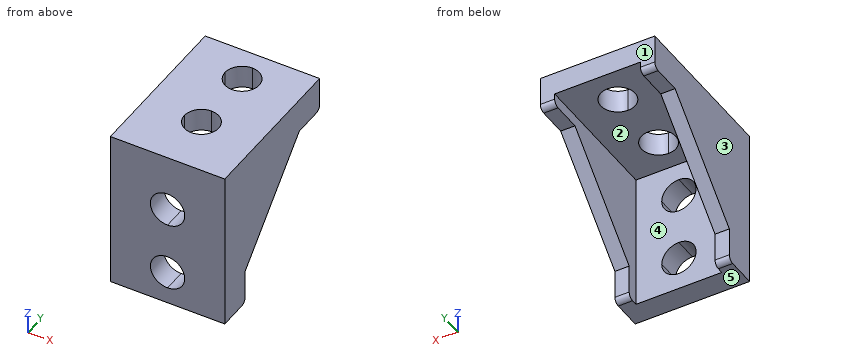
```python
from build123d import *

# Parameters (mm, degrees)
SKETCH1_W               = 17.5
SKETCH1_H               = 16
BOSS_EXTRUDE1_DEPTH     = 6
SKETCH2_W               = 2.5
SKETCH2_H               = 16
BOSS_EXTRUDE2_DEPTH     = 22
BOSS_EXTRUDE3_DEPTH     = 2.5
BOSS_EXTRUDE4_DEPTH     = 6
SKETCH5_W               = 20
SKETCH5_H               = 28
BOSS_EXTRUDE5_DEPTH     = 6
CUT_EXTRUDE1_REACH      = 40.21
SKETCH7_W               = 15
SKETCH7_H               = 22
CUT_EXTRUDE2_REACH      = 40.21
SKETCH9_W               = 15
SKETCH9_H               = 24
CUT_EXTRUDE3_DEPTH      = 45.362146026
CUT_EXTRUDE4_DEPTH      = 39.209946349
CUT_EXTRUDE5_DEPTH      = 41.841155713
BOSS_EXTRUDE6_DEPTH     = 6
BOSS_EXTRUDE7_DEPTH     = 6
BOSS_EXTRUDE8_DEPTH     = 6
BOSS_EXTRUDE9_DEPTH     = 6
FILLET1_R               = 1
SKETCH17_W              = 15
SKETCH17_H              = 24
BOSS_EXTRUDE10_DEPTH    = 4
SKETCH18_W              = 15
SKETCH18_H              = 24
BOSS_EXTRUDE11_DEPTH    = 4
CUT_EXTRUDE6_DEPTH      = 10
CUT_EXTRUDE7_DEPTH      = 10
CUT_EXTRUDE8_DEPTH      = 39.52596527
CUT_EXTRUDE8_DEPTH_BACK = 39.52596527
SKETCH21_W              = 6
SKETCH21_H              = 1.6
CUT_EXTRUDE9_DEPTH      = 39.52596527
CUT_EXTRUDE9_DEPTH_BACK = 39.52596527
SKETCH22_W              = 6
SKETCH22_H              = 1.6


with BuildPart() as part:
    # Sketch1 → Boss-Extrude1 (new body)
    with BuildSketch(Plane.XY):
        with Locations((-1.25, 14)):
            Rectangle(SKETCH1_W, SKETCH1_H)
    extrude(amount=-BOSS_EXTRUDE1_DEPTH)

    # Sketch2 → Boss-Extrude2 (add)
    with BuildSketch(Plane(origin=(0, 0, -6), x_dir=(-1, 0, 0), z_dir=(0, 0, -1))):
        with Locations((8.75, 14)):
            Rectangle(SKETCH2_W, SKETCH2_H)
    extrude(amount=BOSS_EXTRUDE2_DEPTH)

    # Sketch3 → Boss-Extrude3 (add)
    with BuildSketch(Plane(origin=(7.5, 0, 0), x_dir=(0, 0, -1), z_dir=(1, 0, 0))):
        Polygon((6, 22), (22, 6), (0, 6), (0, 22), align=None)
    extrude(amount=BOSS_EXTRUDE3_DEPTH)

    # Sketch4 → Boss-Extrude4 (add)
    with BuildSketch(Plane(origin=(0, 22, 0), x_dir=(-1, 0, 0), z_dir=(0, 1, 0))):
        Polygon((7.5, -6), (-10, -6), (-10, 0), (10, 0), (10, -28), (7.5, -28), align=None)
    extrude(amount=BOSS_EXTRUDE4_DEPTH)

    # Sketch5 → Boss-Extrude5 (add)
    with BuildSketch(Plane.XZ.offset(-6)):
        with Locations((0, -14)):
            Rectangle(SKETCH5_W, SKETCH5_H)
    extrude(amount=BOSS_EXTRUDE5_DEPTH)

    # Sketch7 → Cut-Extrude1 (cut, up to next)
    with BuildSketch(Plane.XY.offset(-4), mode=Mode.PRIVATE) as cut_extrude1_sk1:
        with Locations((0, 17)):
            Rectangle(SKETCH7_W, SKETCH7_H)
    cut_extrude1_tool1 = extrude(cut_extrude1_sk1.sketch, amount=-CUT_EXTRUDE1_REACH, mode=Mode.PRIVATE) & part.part
    add(cut_extrude1_tool1.solids().sort_by_distance((0, 17, -4))[0], mode=Mode.SUBTRACT)

    # Sketch9 → Cut-Extrude2 (cut, up to next)
    with BuildSketch(Plane.XZ.offset(-4), mode=Mode.PRIVATE) as cut_extrude2_sk1:
        with Locations((0, -16)):
            Rectangle(SKETCH9_W, SKETCH9_H)
    cut_extrude2_tool1 = extrude(cut_extrude2_sk1.sketch, amount=-CUT_EXTRUDE2_REACH, mode=Mode.PRIVATE) & part.part
    add(cut_extrude2_tool1.solids().sort_by_distance((0, 4, -16))[0], mode=Mode.SUBTRACT)

    # Sketch10 → Cut-Extrude3 (cut, through all)
    with BuildSketch(Plane.ZY.offset(10)):
        Polygon((-28, 28), (-28, 6), (-22, 6), (-6, 22), (-6, 28), align=None)
    extrude(amount=-CUT_EXTRUDE3_DEPTH, mode=Mode.SUBTRACT)

    # Sketch11 → Cut-Extrude4 (cut, through all)
    with BuildSketch(Plane(origin=(0, 0, -4), x_dir=(-1, 0, 0), z_dir=(0, 0, -1))):
        with BuildLine():
            Line((3.25, 12.5), (3.25, 18))
            ThreePointArc((3.25, 18), (0, 21.25), (-3.25, 18))
            Line((-3.25, 18), (-3.25, 12.5))
            ThreePointArc((-3.25, 12.5), (0, 9.25), (3.25, 12.5))
        make_face()
    extrude(amount=-CUT_EXTRUDE4_DEPTH, mode=Mode.SUBTRACT)

    # Sketch12 → Cut-Extrude5 (cut, through all)
    with BuildSketch(Plane.XZ):
        with BuildLine():
            Line((3.25, -18), (3.25, -12.5))
            ThreePointArc((3.25, -12.5), (0, -9.25), (-3.25, -12.5))
            Line((-3.25, -12.5), (-3.25, -18))
            ThreePointArc((-3.25, -18), (0, -21.25), (3.25, -18))
        make_face()
    extrude(amount=-CUT_EXTRUDE5_DEPTH, mode=Mode.SUBTRACT)

    # Sketch13 → Boss-Extrude6 (add)
    with BuildSketch(Plane(origin=(3, 0, 0), x_dir=(0, 0, -1), z_dir=(1, 0, 0))):
        Polygon((0, 26.5), (-1.6, 24.9), (-1.6, 23.5), (0, 23.5), align=None)
    extrude(amount=-BOSS_EXTRUDE6_DEPTH)

    # Sketch14 → Boss-Extrude7 (add)
    with BuildSketch(Plane(origin=(3, 0, 0), x_dir=(0, 0, -1), z_dir=(1, 0, 0))):
        Polygon((0, 6.5), (-1.6, 4.9), (-1.6, 3.5), (0, 3.5), align=None)
    extrude(amount=-BOSS_EXTRUDE7_DEPTH)

    # Sketch15 → Boss-Extrude8 (add)
    with BuildSketch(Plane(origin=(3, 0, 0), x_dir=(0, 0, -1), z_dir=(1, 0, 0))):
        Polygon((23.5, 0), (23.5, -1.6), (24.9, -1.6), (26.5, 0), align=None)
    extrude(amount=-BOSS_EXTRUDE8_DEPTH)

    # Sketch16 → Boss-Extrude9 (add)
    with BuildSketch(Plane(origin=(3, 0, 0), x_dir=(0, 0, -1), z_dir=(1, 0, 0))):
        Polygon((3.5, 0), (3.5, -1.6), (4.9, -1.6), (6.5, 0), align=None)
    extrude(amount=-BOSS_EXTRUDE9_DEPTH)

    # Fillet1
    fillet1_edges = [part.edges().sort_by_distance(p)[0] for p in [
        (-8.75, 6, -28),
        (8.75, 28, -6),
        (8.75, 6, -28),
        (-8.75, 28, -6),
    ]]
    fillet(fillet1_edges, radius=FILLET1_R)

    # Sketch17 → Boss-Extrude10 (add)
    with BuildSketch(Plane(origin=(0, 4, 0), x_dir=(1, 0, 0), z_dir=(0, 1, 0))):
        with Locations((0, 16)):
            Rectangle(SKETCH17_W, SKETCH17_H)
    extrude(amount=-BOSS_EXTRUDE10_DEPTH)

    # Sketch18 → Boss-Extrude11 (add)
    with BuildSketch(Plane(origin=(0, 0, -4), x_dir=(-1, 0, 0), z_dir=(0, 0, -1))):
        with Locations((0, 16)):
            Rectangle(SKETCH18_W, SKETCH18_H)
    extrude(amount=-BOSS_EXTRUDE11_DEPTH)

    # Sketch20 → Cut-Extrude6 (cut)
    with BuildSketch(Plane(origin=(0, 0, -4), x_dir=(-1, 0, 0), z_dir=(0, 0, -1))):
        with BuildLine():
            ThreePointArc((3, 22), (2.121320344, 24.121320344), (0, 25))
            Line((0, 25), (0, 22))
            Line((0, 22), (0, 19))
            ThreePointArc((0, 19), (2.121320344, 19.878679656), (3, 22))
        make_face()
        with BuildLine():
            Line((0, 22), (0, 25))
            ThreePointArc((0, 25), (-3, 22), (0, 19))
            Line((0, 19), (0, 22))
        make_face()
        with BuildLine():
            ThreePointArc((3, 10), (2.121320344, 12.121320344), (0, 13))
            Line((0, 13), (0, 10))
            Line((0, 10), (0, 7))
            ThreePointArc((0, 7), (2.121320344, 7.878679656), (3, 10))
        make_face()
        with BuildLine():
            Line((0, 10), (0, 13))
            ThreePointArc((0, 13), (-3, 10), (0, 7))
            Line((0, 7), (0, 10))
        make_face()
    extrude(amount=-CUT_EXTRUDE6_DEPTH, mode=Mode.SUBTRACT)

    # Sketch19 → Cut-Extrude7 (cut)
    with BuildSketch(Plane(origin=(0, 4, 0), x_dir=(1, 0, 0), z_dir=(0, 1, 0))):
        with BuildLine():
            Line((0, 19.123546409), (0, 22))
            Line((0, 22), (0, 22.123546409))
            Line((0, 22.123546409), (0, 25.123546409))
            ThreePointArc((0, 25.123546409), (-3, 22.123546409), (0, 19.123546409))
        make_face()
        with BuildLine():
            Line((0, 22.123546409), (0, 22))
            Line((0, 22), (0, 19.123546409))
            ThreePointArc((0, 19.123546409), (2.121320344, 20.002226065), (3, 22.123546409))
            ThreePointArc((3, 22.123546409), (2.121320344, 24.244866752), (0, 25.123546409))
            Line((0, 25.123546409), (0, 22.123546409))
        make_face()
        with BuildLine():
            ThreePointArc((3, 10), (2.121320344, 12.121320344), (0, 13))
            Line((0, 13), (0, 10))
            Line((0, 10), (0, 7))
            ThreePointArc((0, 7), (2.121320344, 7.878679656), (3, 10))
        make_face()
        with BuildLine():
            Line((0, 10), (0, 13))
            ThreePointArc((0, 13), (-3, 10), (0, 7))
            Line((0, 7), (0, 10))
        make_face()
    extrude(amount=-CUT_EXTRUDE7_DEPTH, mode=Mode.SUBTRACT)

    # Sketch21 → Cut-Extrude8 (cut, two sides: drawn at the far end of the back side and taken through both)
    with BuildSketch(Plane.XZ.offset(-3.5).offset(-CUT_EXTRUDE8_DEPTH_BACK)):
        with Locations((0, 0.8)):
            Rectangle(SKETCH21_W, SKETCH21_H)
    extrude(amount=CUT_EXTRUDE8_DEPTH + CUT_EXTRUDE8_DEPTH_BACK, mode=Mode.SUBTRACT)

    # Sketch22 → Cut-Extrude9 (cut, two sides: drawn at the far end of the back side and taken through both)
    with BuildSketch(Plane.XY.offset(-3.5).offset(-CUT_EXTRUDE9_DEPTH_BACK)):
        with Locations((0, -0.8)):
            Rectangle(SKETCH22_W, SKETCH22_H)
    extrude(amount=CUT_EXTRUDE9_DEPTH + CUT_EXTRUDE9_DEPTH_BACK, mode=Mode.SUBTRACT)


solid = part.part
```
Geometry check sheet. Reference: the model listing, model coordinates, mm. Face numbers are marked on the shaded views. A direction names the side the tool comes from. Give positions to 0.01 mm unless a question says otherwise; leave off trailing zeros. Loops run counter-clockwise (first coordinate to the right, second up) from the corner with the lowest first, then second, coordinate; pieces in that order, holes last. Notation, with made-up numbers: M 59,-34.75 L 116,-34.75 A14 ccw 116,-10.75 Z; hole C 76,48 d2. An arc over 180 degrees is marked long. Answer as CSV lines item,"result".
Item 1: Release check for a two-part mould opening along X. For the marked faces 1, 2 and 3 record: pulls with the +X half, pulls with the -X half, needs draft (parallel to the pull), parting line crosses it, or undercut.
Values:
face 1,"needs draft"
face 2,"undercut"
face 3,"pulls with the -X half"
Item 2: Cross-section at B-B on z = -26. Record the cut outline in (x, y), and give its area (3 significant figures).
Values:
outline,"M -10,0 L 10,0 L 10,6 L 7.5,6 L 7.5,4 L -7.5,4 L -7.5,6 L -10,6 Z"
area,"90.0 mm²"
Item 3: Access from +Z, -Z, +X, -X, +Y, -Y to the whole of each face (thin tool, end or side, straight path). Record for the marked faces 4 and 5.
Values:
face 4,"-Z, +Y"
face 5,"-Z, +X, -X, +Y, -Y"
Item 4: Cross-section at A-A on y = 2. Record the cut outline in (x, z), and give its area (3 significant figures).
Values:
outline,"M -10,-28 L 10,-28 L 10,0 L -10,0 Z; hole C 0,-22.12 d6; hole C 0,-10 d6"
area,"503 mm²"
Item 5: Material ranges on line 1 (X direction, y = 4.25, z = -26.25); line 2 (Z direction, x = 1.75, y = 12.75); line 3 (Y direction, x = -6.5, z = -14), recorded low to high.
Values:
line 1,"x = -10 to -7.5, 7.5 to 10"
line 2,"z = -4 to 0"
line 3,"y = 0 to 4"
Item 6: Cross-section at D-D on y = 24.5. Record the cut outline in (x, z).
Values:
outline,"M -10,-6 L -7.5,-6 L -7.5,-4 L -1.66,-4 L -1.66,0 L -10,0 Z; M 1.66,-4 L 7.5,-4 L 7.5,-6 L 10,-6 L 10,0 L 1.66,0 Z"
Item 7: Depth check by flat-ended pin: P1, Ø2, axis at x = -8.5, y = 23.5, coming from the -Z side; P2, Ø1.2, axis at x = 8.5, z = -24.5, coming from the +Y side; P3, Ø1.5, axis at x = 6.5, y = 7, coming from the +Z side; P4, Ø1, axis at x = -0.5, y = 13.5, coming from the -Z side. Enter the tip coordinate at first touch or a pass-through.
Values:
P1,"stops at z = -6"
P2,"stops at y = 6"
P3,"stops at z = 0"
P4,"stops at z = -4"
Item 8: Cross-section at C-C on x = 2.25. Record the cut outline in (y, z), and give its area (3 significant figures).
Values:
outline,"M 0,-28 L 4,-28 L 4,-24.11 L 0,-24.11 Z; M 0,-20.14 L 4,-20.14 L 4,-11.98 L 0,-11.98 Z; M 0,-8.02 L 4,-8.02 L 4,-4 L 8.02,-4 L 8.02,0 L 0,0 Z; M 11.98,-4 L 20.02,-4 L 20.02,0 L 11.98,0 Z; M 23.98,-4 L 28,-4 L 28,0 L 23.98,0 Z"
area,"145 mm²"
